Could you check a few things on this model? Use its own coordinates, in mm. Give positions to 0.01 mm unless a question says otherwise; leave off trailing zeros. Loops run counter-clockwise (first coordinate to the right, second up) from the corner with the lowest first, then second, coordinate; pieces in that order, holes last. Notation, with made-up numbers: M 31,0.5 L 39,0.5 A8 cw 39,6.5 Z; hole C 13,60.25 d4. An arc over 180 degrees is marked long. Use a Markdown table: item, result. Add a question column.
1) If I drill on line 1 along X through (y, z) = (-0.2, 4.5); line 2 along Z through (x, y) = (-2.75, -0.85); line 3 along X through (y, z) = (-0.2, -29.5), over which ranges is the centre line in solid material (lowest first)? Write a range as [from, to].
2) Suppose I cut it at A-A on z = -12.7. List the corners of the cut face in (x, y) for me.
3) Will these pins go through, and if not, where does the flat tip stop? pin 1 Ø0.9 at (y, z) = (-2, -27.5) entering from +X; pin 2 Ø0.9 at (x, y) = (-1, -2) entering from +Z.
4) Suppose I cut it at C-C on x = -8.5. List the corners of the cut face in (y, z) for me, and give its area (3 significant figures).
5) Suppose I cut it at B-B on y = -0.45. List the corners of the cut face in (x, z) for me, and give its area (3 significant figures).
```python
from build123d import *

# Parameters (mm, degrees)
F0_R     = 1.651
F1_DEPTH = 3.0226


with BuildPart() as f1:
    # F0 (on Front) → F1 (new body)
    with BuildSketch(Plane.XZ):
        Polygon((0, -25.4), (0, 0), (-2.928276, 0), (-2.928276, 6.35), (-15.628276, 6.35), (-15.628276, -31.75), (-2.9718, -31.75), (-2.9718, -25.4), align=None)
        with Locations((-9.278276, -25.4)):
            Circle(F0_R, mode=Mode.SUBTRACT)
        with Locations((-9.278276, -12.7)):
            Circle(F0_R, mode=Mode.SUBTRACT)
        with Locations((-9.278276, 0)):
            Circle(F0_R, mode=Mode.SUBTRACT)
    extrude(amount=F1_DEPTH)


solid = f1.part
```
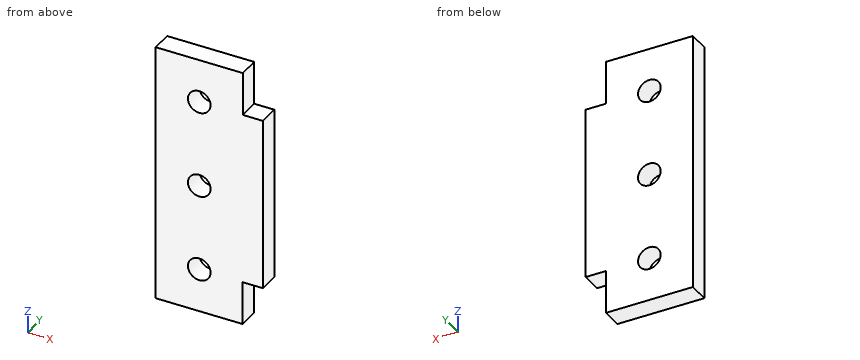
Answer block:
| question | item | result |
|---|---|---|
| 1 | line 1 | x = [-15.63, -2.93] |
| 1 | line 2 | z = [-25.4, 0] |
| 1 | line 3 | x = [-15.63, -2.97] |
| 2 | outline | M -15.63,-3.02 L -10.93,-3.02 L -10.93,0 L -15.63,0 Z; M -7.63,-3.02 L 0,-3.02 L 0,0 L -7.63,0 Z |
| 3 | pin 1 | stops at x = -2.97 |
| 3 | pin 2 | stops at z = 0 |
| 4 | outline | M -3.02,-31.75 L 0,-31.75 L 0,-26.86 L -3.02,-26.86 Z; M -3.02,-23.94 L 0,-23.94 L 0,-14.16 L -3.02,-14.16 Z; M -3.02,-11.24 L 0,-11.24 L 0,-1.46 L -3.02,-1.46 Z; M -3.02,1.46 L 0,1.46 L 0,6.35 L -3.02,6.35 Z |
| 4 | area | 88.8 mm^2 |
| 5 | outline | M -15.63,-31.75 L -2.97,-31.75 L -2.97,-25.4 L 0,-25.4 L 0,0 L -2.93,0 L -2.93,6.35 L -15.63,6.35 Z; hole C -9.28,-25.4 d3.3; hole C -9.28,-12.7 d3.3; hole C -9.28,0 d3.3 |
| 5 | area | 532 mm^2 |
